The listing builds one solid part. Answer for the finished solid, in the listing's coordinates (mm). A direction names the side the tool comes from. Round coordinates to 2 decimals unless told otherwise and drop trailing zeros. Write each loop counter-clockwise with the first axis right and the second up, starting at its lowest first coordinate (ties: lowest second). Pieces come first, ordered by that corner, then holes.
(1) For faces 4 (the face through (13.583, -18.966, 0.493)), 5 (the face through (13, -19, 0)), 6 (the face through (6.278, -9.353, 0.493)), determine the directions among +Z, -Z, +X, -X, +Y, -Y from which every point of the face is accessible in a straight line to the end or side of a thin tool.
(2) A cutting plane is placed at B-B, the plane z = 0.25. Give the number of separate pieces and of enclosed holes in the cut face, and give its area (3 significant figures).
(3) A cutting plane is placed at C-C, the plane y = -35.5. Give the vertices of the cut face in (x, z), and give its area (3 significant figures).
(4) A cutting plane is placed at A-A, the plane y = 0. Give the vertices of the cut face in (x, z), and give its area (3 significant figures).
(5) Find the intervals of material crossed by probe 1 along Y at (x, z) = (4.5, 0.85); probe 2 along X at (y, z) = (-16, 0.6); probe 3 along X at (y, z) = (-40, 0.85), in increasing order.
(6) A cutting plane is placed at D-D, the plane y = -50. Give the vertices of the cut face in (x, z), and give its area (3 significant figures).
(7) The mould has two halves that part along X. Classify faces 1 (the face through (13, -19, 1)), 2 (the face through (23.6, -36.45, 0.49)), 3 (the face through (12.568, 9.658, 0.493)): +X half, -X half, draft (parallel to the pull), parting line (faces both ways), or undercut.
from build123d import *

# Parameters (mm, degrees)
SKETCH1_R           = 1
SKETCH1_R_2         = 2.25
SKETCH1_R_3         = 0.998074624
BOSS_EXTRUDE2_DEPTH = 1


with BuildPart() as part:
    # Sketch1 → Boss-Extrude2 (new body)
    with BuildSketch(Plane.XY):
        with BuildLine():
            Line((5.146977165, -5.612602972), (7.44171219, -13.199988708))
            ThreePointArc((7.44171219, -13.199988708), (7.439945118, -13.784749424), (7.111476, -14.268543033))
            ThreePointArc((7.111476, -14.268543033), (5.923924569, -18.62818009), (9.697794763, -21.113057841))
            ThreePointArc((9.697794763, -21.113057841), (10.380528536, -21.341854348), (10.732574986, -21.969975788))
            ThreePointArc((10.732574986, -21.969975788), (10.79176698, -22.393908793), (10.847713449, -22.818282305))
            ThreePointArc((10.847713449, -22.818282305), (11.790244876, -24.335347863), (11.163215941, -26.007678007))
            ThreePointArc((11.163215941, -26.007678007), (10.570290463, -27.483765064), (11.290805177, -28.901951289))
            ThreePointArc((11.290805177, -28.901951289), (11.931562756, -30.214937196), (11.277042335, -31.52111685))
            ThreePointArc((11.277042335, -31.52111685), (10.500432467, -32.761716535), (11.145287396, -34.075631519))
            ThreePointArc((11.145287396, -34.075631519), (11.711049486, -35.240414103), (10.937199745, -36.278663489))
            ThreePointArc((10.937199745, -36.278663489), (10.185540032, -37.265502357), (10.650830557, -38.415436269))
            ThreePointArc((10.650830557, -38.415436269), (11.153884573, -39.735845823), (10.230304321, -40.805212107))
            ThreePointArc((10.230304321, -40.805212107), (9.263580844, -41.700908083), (9.768401259, -42.918274877))
            ThreePointArc((9.768401259, -42.918274877), (10.29278617, -44.215864041), (9.202326649, -45.093141196))
            ThreePointArc((9.202326649, -45.093141196), (8.144843355, -45.909982105), (8.571180325, -47.176369398))
            ThreePointArc((8.571180325, -47.176369398), (8.845608938, -48.309992252), (7.932024848, -49.035096348))
            ThreePointArc((7.932024848, -49.035096348), (7.054134874, -49.652663659), (7.297145805, -50.698142438))
            ThreePointArc((7.297145805, -50.698142438), (7.486031135, -51.627523472), (6.693279806, -52.148073283))
            ThreePointArc((6.693279806, -52.148073283), (5.736341709, -52.667939714), (5.979078831, -53.729575393))
            ThreePointArc((5.979078831, -53.729575393), (6.146574337, -54.831276595), (5.172832259, -55.373149872))
            ThreePointArc((5.172832259, -55.373149872), (4.397991341, -55.805643097), (4.477975588, -56.689402883))
            ThreePointArc((4.477975588, -56.689402883), (4.477842946, -57.805544451), (3.519463877, -58.377629741))
            ThreePointArc((3.519463877, -58.377629741), (2.763689302, -58.882818754), (2.639049746, -59.78330536))
            ThreePointArc((2.639049746, -59.78330536), (2.762025793, -60.669472955), (2.167842085, -61.338324084))
            ThreePointArc((2.167842085, -61.338324084), (1.808869059, -61.604258533), (1.601521968, -61.999973009))
            ThreePointArc((1.601521968, -61.999973009), (1.407536389, -62.888842845), (1.289722883, -63.790973638))
            ThreePointArc((1.289722883, -63.790973638), (1.548602642, -64.553775113), (2.285909866, -64.878217524))
            Line((2.285909866, -64.878217524), (4.16607409, -64.878217524))
            ThreePointArc((4.16607409, -64.878217524), (4.576078061, -64.790301261), (4.913989999, -64.54201101))
            Line((4.913989999, -64.54201101), (19.858030846, -47.704114694))
            ThreePointArc((19.858030846, -47.704114694), (21.299586827, -45.585122466), (22.155211357, -43.169316519))
            Line((22.155211357, -43.169316519), (25.087470282, -29.538838187))
            ThreePointArc((25.087470282, -29.538838187), (25.281255234, -26.663292069), (24.646889926, -23.851904734))
            Line((24.646889926, -23.851904734), (16.800568019, -3.412304746))
            ThreePointArc((16.800568019, -3.412304746), (16.953922391, -3.093842948), (17.092102067, -2.768509492))
            Line((17.092102067, -2.768509492), (18.525386899, -3.188095126))
            ThreePointArc((18.525386899, -3.188095126), (19.785478354, -2.423398267), (18.979727986, -1.189154327))
            Line((18.979727986, -1.189154327), (17.575945858, -0.827918039))
            ThreePointArc((17.575945858, -0.827918039), (17.62064019, 0.130893048), (17.54251106, 1.087560245))
            Line((17.54251106, 1.087560245), (18.993564953, 1.440830843))
            ThreePointArc((18.993564953, 1.440830843), (19.702487734, 2.733123476), (18.387565476, 3.399134899))
            Line((18.387565476, 3.399134899), (16.991236349, 3.010083636))
            ThreePointArc((16.991236349, 3.010083636), (16.550537232, 3.862785562), (16.004541822, 4.652219092))
            Line((16.004541822, 4.652219092), (17.084556057, 5.68368735))
            ThreePointArc((17.084556057, 5.68368735), (17.052354878, 7.157306991), (15.580593087, 7.076628673))
            Line((15.580593087, 7.076628673), (14.565862222, 6.041535833))
            ThreePointArc((14.565862222, 6.041535833), (13.757854628, 6.559647804), (12.890291968, 6.97031959))
            Line((12.890291968, 6.97031959), (13.309877602, 8.403604423))
            ThreePointArc((13.309877602, 8.403604423), (12.545180743, 9.663695877), (11.310936803, 8.857945509))
            Line((11.310936803, 8.857945509), (10.949700516, 7.454163382))
            ThreePointArc((10.949700516, 7.454163382), (9.990889428, 7.498857714), (9.034222232, 7.420728584))
            Line((9.034222232, 7.420728584), (8.680951634, 8.871782476))
            ThreePointArc((8.680951634, 8.871782476), (7.388659, 9.580705258), (6.722647578, 8.265783))
            Line((6.722647578, 8.265783), (7.11169884, 6.869453872))
            ThreePointArc((7.11169884, 6.869453872), (6.258996915, 6.428754755), (5.469563385, 5.882759346))
            Line((5.469563385, 5.882759346), (4.438095126, 6.96277358))
            ThreePointArc((4.438095126, 6.96277358), (2.964475486, 6.930572401), (3.045153803, 5.45881061))
            Line((3.045153803, 5.45881061), (4.080246644, 4.444079745))
            ThreePointArc((4.080246644, 4.444079745), (3.562134673, 3.636072152), (3.151462886, 2.768509492))
            Line((3.151462886, 2.768509492), (1.718178054, 3.188095126))
            ThreePointArc((1.718178054, 3.188095126), (0.458086599, 2.423398267), (1.263836967, 1.189154327))
            Line((1.263836967, 1.189154327), (2.667619095, 0.827918039))
            ThreePointArc((2.667619095, 0.827918039), (2.622924763, -0.130893048), (2.701053893, -1.087560245))
            Line((2.701053893, -1.087560245), (1.25, -1.440830843))
            ThreePointArc((1.25, -1.440830843), (0.541077219, -2.733123476), (1.855999477, -3.399134899))
            Line((1.855999477, -3.399134899), (3.252328604, -3.010083636))
            ThreePointArc((3.252328604, -3.010083636), (4.058376204, -4.414193514), (5.146977165, -5.612602972))
        make_face()
        with Locations((10.121782476, 0)):
            Circle(SKETCH1_R, mode=Mode.SUBTRACT)
        with Locations((15.627966379, -9.260281964)):
            Circle(SKETCH1_R_2, mode=Mode.SUBTRACT)
        with Locations((9.121782476, -17.526259213)):
            Circle(SKETCH1_R_3, mode=Mode.SUBTRACT)
        with Locations((22, -26.49969455)):
            Circle(SKETCH1_R, mode=Mode.SUBTRACT)
        with Locations((21.5, -33.166361217)):
            Circle(SKETCH1_R, mode=Mode.SUBTRACT)
        with Locations((18.474150388, -39.833027883)):
            Circle(SKETCH1_R, mode=Mode.SUBTRACT)
        with Locations((17.55481685, -46.49969455)):
            Circle(SKETCH1_R, mode=Mode.SUBTRACT)
        with BuildLine():
            Line((14.500290742, -21.375988683), (12.638736062, -16.487053928))
            ThreePointArc((12.638736062, -16.487053928), (13.337027802, -14.929994394), (14.894087335, -15.628286133))
            Line((14.894087335, -15.628286133), (16.755642015, -20.517220889))
            ThreePointArc((16.755642015, -20.517220889), (16.057350276, -22.074280422), (14.500290742, -21.375988683))
        make_face(mode=Mode.SUBTRACT)
    extrude(amount=BOSS_EXTRUDE2_DEPTH)


solid = part.part
Solutions:
1. face 4: +Z, -Z
1. face 5: -Z, +X, -X, +Y, -Y
1. face 6: +Z, -Z, -X
2. separate pieces: 1
2. enclosed holes: 8
2. area: 848 mm2
3. outline: (11.66, 0) - (23.81, 0) - (23.81, 1) - (11.66, 1) - close
3. area: 12.1 mm2
4. outline: (2.62, 0) - (9.12, 0) - (9.12, 1) - (2.62, 1) - close; (11.12, 0) - (17.62, 0) - (17.62, 1) - (11.12, 1) - close
4. area: 13.0 mm2
5. probe 1: y = -64.82 to -57.76, -56.73 to -55.66, -4.96 to 6.9
5. probe 2: x = 5.89 to 12.56, 15.04 to 21.63
5. probe 3: x = 11.08 to 17.49, 19.46 to 22.84
6. outline: (6.99, 0) - (17.82, 0) - (17.82, 1) - (6.99, 1) - close
6. area: 10.8 mm2
7. face 1: draft
7. face 2: +X half
7. face 3: undercut
